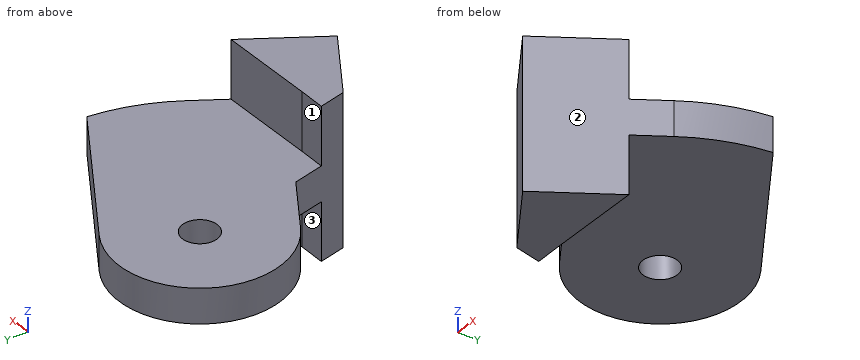
Autodesk Inventor part; units mm, degrees
ref_plane "Work Plane2" through (162.2, -27.5, -5) normal (0, 0, -1) x (0, 1, 0)
ref_plane "YZ Plane" through (0, 0, 0) normal (1, 0, 0) x (0, 1, 0)
ref_plane "XZ Plane" through (0, 0, 0) normal (0, 1, 0) x (-1, 0, 0)
ref_plane "Work Plane1" through (0, 0, 0) normal (0, 0, 1) x (1, 0, 0)
sketch "Sketch1" plane through (0, 0, 0) normal (0, 0, 1) x (1, 0, 0)
  circle A0 centre (178.666376, -16.397041) radius 1.5
  line L0 (201.424818, -12.080439) -> (122.055329, -134.544275)
  line L1 (192.303309, -25.235213) -> (190.399763, -28.172305)
  arc A1 (180.569922, -13.459949) -> (176.76283, -19.334134) centre (178.666376, -16.397041) ccw
  line L2 (182.927065, -27.5) -> (174.859284, -22.271227)
  arc A2 (182.473468, -10.522856) -> (174.859284, -22.271227) centre (178.666376, -16.397041) ccw
  line L3 (226.007006, -27.5) -> (182.061376, -27.5)
  line L4 (203.888132, -20.231027) -> (184.377014, -7.585764)
  line L5 (182.473468, -10.522856) -> (194.780372, -18.499029)
  line L6 (180.718486, -30.239399) -> (187.012256, -34.318426)
  arc A3 (192.303309, -25.235213) -> (194.780372, -18.499029) centre (178.666376, -16.397041) ccw
  line L7 (182.622032, -27.302306) -> (180.718486, -30.239399)
  line L8 (192.303309, -25.235213) -> (186.592671, -34.046491)
  point P0 (0, 0)
  point P1 (182.493905, -27.5)
  dimension "d0" = 0.5
  dimension "d1" = 7
extrude "Extrusion1" add sketch "Sketch1" along normal blind 3 contours L3 L2 A2 L5 A3 L1 | L1 L8 L6 L7 L3 | L3 L7 L2
sketch "Sketch2" plane through (0, 0, 0) normal (0, 0, -1) x (-1, 0, 0)
  line L0 (-113.222122, -27.5) -> (-151.8, -27.5)
  line L1 (-182.622032, -27.302306) -> (-180.718486, -30.239399)
  line L2 (-180.718486, -30.239399) -> (-186.592671, -34.046491)
  line L3 (-121.635744, -134.27234) -> (-201.005233, -11.808504)
  line L4 (-182.493905, -27.5) -> (-182.493905, -28)
  line L5 (-182.493905, -28) -> (-182.265706, -27.852103)
  line L6 (-182.622032, -27.302306) -> (-180.718486, -30.239399)
  line L7 (-182.493905, -28) -> (-182.169853, -28)
  line L8 (-182.169853, -28) -> (-190.607288, -27.852103)
  point P0 (0, 0)
  point P1 (-182.493905, -27.99432)
  dimension "d10" = 0.5
ref_plane "Work Plane2" through (162.2, -27.5, -5) normal (0, 0, -1) x (0, 1, 0)
extrude "Extrusion2" add sketch "Sketch2" along normal up to surface (5 mm away) contours L4 L7 L1 L2 L3 L8
sketch "Sketch3" plane through (0, 0, 3) normal (0, 0, 1) x (1, 0, 0)
  line L0 (190.607288, -27.852103) -> (182.493905, -27.99432)
  line L1 (186.592671, -34.046491) -> (190.607288, -27.852103)
  line L2 (180.718486, -30.239399) -> (186.592671, -34.046491)
  line L3 (182.169853, -28) -> (180.718486, -30.239399)
  line L4 (182.493905, -28) -> (182.169853, -28)
  line L5 (182.493905, -27.99432) -> (182.493905, -28)
  point P0 (0, 0)
extrude "Extrusion3" add sketch "Sketch3" along normal blind 5
chamfer "Chamfer1" distance 3.5 angle 45 1 edges at (182.622, -27.3023, 1.5)
properties part number "Lock1_3DPrint"
Geometry check sheet. Reference: the model listing, model coordinates, mm. Face numbers are marked on the shaded views. A direction names the side the tool comes from. Give positions to 0.01 mm unless a question says otherwise; leave off trailing zeros. Loops run counter-clockwise (first coordinate to the right, second up) from the corner with the lowest first, then second, coordinate; pieces in that order, holes last. Notation, with made-up numbers: (-21.5, 21.25) -> (12.5, 21.25) arc R33 cw to (12.5, 52.25) -> close; hole circle Ø7 at (-1, 36.25). An arc over 180 degrees is marked (long way). Answer in a Markdown table with one row per item. Add a question column.
1) Material ranges on probe 1 along Z at (x, y) = (187.25, -23.5); probe 2 along Y at (x, z) = (179.5, 2.5); probe 3 along X at (y, z) = (-15.75, 1.75), recorded low to high. Write a range as from..to.
2) Set-up check for the marked faces 1, 2 and 3: record each of +Z, -Z, +X, -X, +Y, -Y from which the full face is reachable in a straight line by a thin tool's end or side.
3) Cross-section at A-A on x = 178. Record the boundary of the cut face in (y, z).
4) Cross-section at B-B on z = 0.75. Record the boundary of the cut face in (x, y).
5) Gauge pin test, flat ends, axial feed: P1, Ø5.5, axis at x = 181, y = -17.5, coming from the -Z side; P2, Ø2, axis at x = 191.5, y = -19, coming from the +Z side; P3, Ø1.1, axis at x = 181.5, z = -3.5, coming from the +Y side. Record the tip position at first contact, or that the pin passes through.
6) Cross-section at C-C on y = -17. Record the boundary of the cut face in (x, z), and give its area (3 significant figures).
Outcome:
| question | item | result |
|---|---|---|
| 1 | probe 1 | z = 0..3 |
| 1 | probe 2 | y = -25.28..-17.64, -15.15..-9.45 |
| 1 | probe 3 | x = 171.7..177.31, 180.02..190.54 |
| 2 | face 1 | +Z, -X, +Y |
| 2 | face 2 | +Z, -Z, +X, -Y |
| 2 | face 3 | -Z, -X, +Y |
| 3 | outline | (-24.31, 0) -> (-17.74, 0) -> (-17.74, 3) -> (-24.31, 3) -> close; (-15.05, 0) -> (-9.43, 0) -> (-9.43, 3) -> (-15.05, 3) -> close |
| 4 | outline | (174.86, -22.27) -> (179.68, -25.4) -> (180.72, -30.24) -> (186.59, -34.05) -> (192.3, -25.24) arc R16.25 ccw to (194.78, -18.5) -> (182.47, -10.52) arc R7 ccw to start; hole circle Ø3 at (178.67, -16.4) |
| 5 | P1 | stops at z = 0 |
| 5 | P2 | stops at z = 3 |
| 5 | P3 | stops at y = -28 |
| 6 | outline | (171.69, 0) -> (177.29, 0) -> (177.29, 3) -> (171.69, 3) -> close; (180.04, 0) -> (192.47, 0) -> (192.47, 3) -> (180.04, 3) -> close |
| 6 | area | 54.1 mm^2 |
